The model under review builds one solid part; all positions refer to its coordinate system, in mm. A direction names the side the tool comes from. Coordinates: 2 decimals unless noted, no trailing zeros. Loops run counter-clockwise (first coordinate to the right, second up) from the corner with the lowest first, then second, coordinate; pieces in that order, holes last. Notation, with made-up numbers: (3, 25) - (20, 25) arc R21 ccw to (20, 34) - close; hole circle Ø7 at (3.5, -9.75). An arc over 180 degrees is marked (long way). Use a Markdown table: item, result. Add a question column.
1) For faces 4 (the flat face through (20, -3, 24)), 5 (the flat face through (0, -14, 22)), list the 3-axis set-ups (+Z, -Z, +X, -X, +Y, -Y) from which the entire face can be reached by the end or side of a thin tool; tool diameter is ignored.
2) To check wall thickness, follow L1, parallel to X at y = -19, z = 40; L2, parallel to Z at x = 3.9, y = -19.05; L3, parallel to Y at x = 24, z = 40. State the ranges of each line that lie inside material, in increasing order. Write a range as [from, to].
3) Clearance check with flat-ended pins moving along their axes: pin 1 (8 mm diameter, centred on x = 19, z = 24.5, fed in from +Y); pin 2 (11.5 mm diameter, centred on x = 33, z = 14, fed in from +Y); pin 3 (13.5 mm diameter, centred on x = 24.05, y = -19.05, fed in from -Z); pin 4 (15.5 mm diameter, centred on y = -20.5, z = 21, fed in from +X). State where each tip first meets the part, or that it passes through.
4) The part is to be moulded in two halves that separate along Y. For faces 1 (the flat face through (16, 0, 27)), 2 (the flat face through (3, -18, 0)), 3 (the flat face through (20, -34.1, 24)), say which applies: pulls with the +Y half, pulls with the -Y half, needs draft (parallel to the pull), parting line crosses it, or undercut.
5) Add section D-D, the plane z = 34.5. Give the boundary of the cut face in (x, y), and give its area (4 significant figures).
6) Add section A-A, the plane x = 24.05. Give the boundary of the cut face in (y, z).
7) Add section B-B, the plane z = 19.05. Give the boundary of the cut face in (x, y).
8) Add section C-C, the plane y = -19.05. Give the boundary of the cut face in (x, z), and give its area (3 significant figures).
```python
from build123d import *

# Parameters (mm, degrees)
PAD001_DEPTH    = 37.1
SKETCH_R        = 4.25
POCKET_DEPTH    = 43.101
SKETCH002_R     = 4.25
POCKET001_DEPTH = 43.101
PAD_DEPTH       = 3
PAD002_DEPTH    = 3


with BuildPart() as part:
    # Sketch001 → Pad001 (new body)
    with BuildSketch(Plane.XZ):
        with BuildLine():
            Line((1, 43.1), (42.1, 43.1))
            ThreePointArc((43.1, 42.1), (42.807107, 42.807107), (42.1, 43.1))
            Line((43.1, 38.1), (43.1, 42.1))
            Line((43.1, 38.1), (6, 38.1))
            ThreePointArc((6, 38.1), (5.292893, 37.807107), (5, 37.1))
            Line((5, 37.1), (5, 0))
            Line((1, 0), (5, 0))
            ThreePointArc((0, 1), (0.292893, 0.292893), (1, 0))
            Line((0, 42.1), (0, 1))
            ThreePointArc((1, 43.1), (0.292893, 42.807107), (0, 42.1))
        make_face()
    extrude(amount=PAD001_DEPTH)

    # Sketch → Pocket (cut, through all)
    with BuildSketch(Plane.XY):
        with Locations((24.05, -19.05)):
            Circle(SKETCH_R)
    extrude(amount=POCKET_DEPTH, mode=Mode.SUBTRACT)

    # Sketch002 → Pocket001 (cut, through all)
    with BuildSketch(Plane.YZ):
        with Locations((-19.05, 19.05)):
            Circle(SKETCH002_R)
    extrude(amount=POCKET001_DEPTH, mode=Mode.SUBTRACT)

    # Sketch003 → Pad (join)
    with BuildSketch(Plane.XZ):
        Polygon((5, 0), (43.1, 38.1), (5, 38.1), align=None)
    extrude(amount=PAD_DEPTH)

    # Sketch004 → Pad002 (join)
    with BuildSketch(Plane.XZ.offset(34.1)):
        Polygon((5, 0), (43.1, 38.1), (5, 38.1), align=None)
    extrude(amount=PAD002_DEPTH)


solid = part.part
```
From the geometry:
| question | item | result |
|---|---|---|
| 1 | face 4 | -Z, +X |
| 1 | face 5 | +Z, -Z, -X, +Y, -Y |
| 2 | L1 | x = [0, 19.8], [28.3, 43.1] |
| 2 | L2 | z = [0, 14.8], [23.3, 43.1] |
| 2 | L3 | y = [-37.1, -23.3], [-14.8, 0] |
| 3 | pin 1 | stops at y = 0 |
| 3 | pin 2 | passes through |
| 3 | pin 3 | stops at z = 38.1 |
| 3 | pin 4 | stops at x = 5 |
| 4 | face 1 | pulls with the +Y half |
| 4 | face 2 | needs draft |
| 4 | face 3 | undercut |
| 5 | outline | (0, -37.1) - (39.5, -37.1) - (39.5, -34.1) - (5, -34.1) - (5, -3) - (39.5, -3) - (39.5, 0) - (0, 0) - close |
| 5 | area | 392.5 mm^2 |
| 6 | outline | (-37.1, 19.05) - (-34.1, 19.05) - (-34.1, 38.1) - (-23.3, 38.1) - (-23.3, 43.1) - (-37.1, 43.1) - close; (-14.8, 38.1) - (-3, 38.1) - (-3, 19.05) - (0, 19.05) - (0, 43.1) - (-14.8, 43.1) - close |
| 7 | outline | (0, -37.1) - (24.05, -37.1) - (24.05, -34.1) - (5, -34.1) - (5, -23.3) - (0, -23.3) - close; (0, -14.8) - (5, -14.8) - (5, -3) - (24.05, -3) - (24.05, 0) - (0, 0) - close |
| 8 | outline | (0, 1) arc R1 ccw to (1, 0) - (5, 0) - (5, 14.8) - (0, 14.8) - close; (0, 23.3) - (5, 23.3) - (5, 37.1) arc R1 cw to (6, 38.1) - (19.8, 38.1) - (19.8, 43.1) - (1, 43.1) arc R1 ccw to (0, 42.1) - close; (28.3, 38.1) - (43.1, 38.1) - (43.1, 42.1) arc R1 ccw to (42.1, 43.1) - (28.3, 43.1) - close |
| 8 | area | 321 mm^2 |
